from build123d import *

# Parameters (mm, degrees)
BOX002_W               = 20
BOX002_H               = 5
BOX002_DEPTH           = 10
BOX_W                  = 22.7
BOX_H                  = 12.6
BOX_DEPTH              = 17
BOX001_W               = 35
BOX001_H               = 15
BOX001_DEPTH           = 17
CUT_PLACEMENT_ANGLE    = 90
CYLINDER002_R          = 2.475
CYLINDER002_DEPTH      = 22.9
CYLINDER001_R          = 6.55
CYLINDER001_DEPTH      = 50
CUBE001_W              = 3.45
CUBE001_H              = 7.11
CUBE001_DEPTH          = 11.11
CUBE_W                 = 8.25
CUBE_H                 = 11.91
CUBE_DEPTH             = 12.91
CYLINDER_R             = 11.45
CYLINDER_DEPTH         = 45
FUSION_PLACEMENT_ANGLE = 90


with BuildPart() as cube002:
    # Box002 → Box002 (new body)
    with BuildSketch(Plane(origin=(-30, -2.5, -1), x_dir=(1, 0, 0), z_dir=(0, 0, 1))):
        with Locations((10, 2.5)):
            Rectangle(BOX002_W, BOX002_H)
    extrude(amount=BOX002_DEPTH)


with BuildPart() as cube:
    # Box → Box (new body)
    with BuildSketch(Plane.XY.offset(1)):
        with Locations((11.35, 6.3)):
            Rectangle(BOX_W, BOX_H)
    extrude(amount=BOX_DEPTH)


with BuildPart() as cut001:
    # Box001 → Box001 (new body)
    with BuildSketch(Plane(origin=(-6, -1, 0), x_dir=(1, 0, 0), z_dir=(0, 0, 1))):
        with Locations((17.5, 7.5)):
            Rectangle(BOX001_W, BOX001_H)
    extrude(amount=BOX001_DEPTH)

    # Cut: cut Cube
    add(cube.part, mode=Mode.SUBTRACT)


with BuildPart() as cut001_1:
    # Cut placement: moved
    add(cut001.part.moved(Location((-11, -6, 6))).rotate(Axis((-11, -6, 6), (0, -1, 0)), CUT_PLACEMENT_ANGLE))

    # Cut001: cut Cube002
    add(cube002.part, mode=Mode.SUBTRACT)


with BuildPart() as cylinder002:
    # cylinder002 → cylinder002 (new body)
    with BuildSketch(Plane(origin=(0, 0, 6.825), x_dir=(0, 0, -1), z_dir=(1, 0, 0))):
        Circle(CYLINDER002_R)
    extrude(amount=CYLINDER002_DEPTH)


with BuildPart() as union001:
    # cylinder001 → cylinder001 (new body)
    with BuildSketch(Plane.XY.offset(-1)):
        Circle(CYLINDER001_R)
    extrude(amount=CYLINDER001_DEPTH)

    # union001: union cylinder002
    add(cylinder002.part)


with BuildPart() as cube001:
    # cube001 → cube001 (new body)
    with BuildSketch(Plane(origin=(-1.725, -3.555, -4.6), x_dir=(1, 0, 0), z_dir=(0, 0, 1))):
        with Locations((1.725, 3.555)):
            Rectangle(CUBE001_W, CUBE001_H)
    extrude(amount=CUBE001_DEPTH)


with BuildPart() as difference:
    # cube → cube (new body)
    with BuildSketch(Plane(origin=(-4.125, -5.955, -6.455), x_dir=(1, 0, 0), z_dir=(0, 0, 1))):
        with Locations((4.125, 5.955)):
            Rectangle(CUBE_W, CUBE_H)
    extrude(amount=CUBE_DEPTH)

    # difference: cut cube001
    add(cube001.part, mode=Mode.SUBTRACT)


with BuildPart() as difference_1:
    # difference placement: moved
    add(difference.part.moved(Location((13.95, 0, 6.425))))


with BuildPart() as motor_holder:
    # cylinder → cylinder (new body)
    with BuildSketch(Plane.XY):
        Circle(CYLINDER_R)
    extrude(amount=CYLINDER_DEPTH)

    # union: union difference
    add(difference_1.part)

    # difference001: cut union001
    add(union001.part, mode=Mode.SUBTRACT)

    # Fusion: union Cut001
    add(cut001_1.part)


with BuildPart() as motor_holder_1:
    # Fusion placement: moved
    add(motor_holder.part.moved(Location((-21, 50, 0))).rotate(Axis((-21, 50, 0), (0, 0, 1)), FUSION_PLACEMENT_ANGLE))


solid = motor_holder_1.part
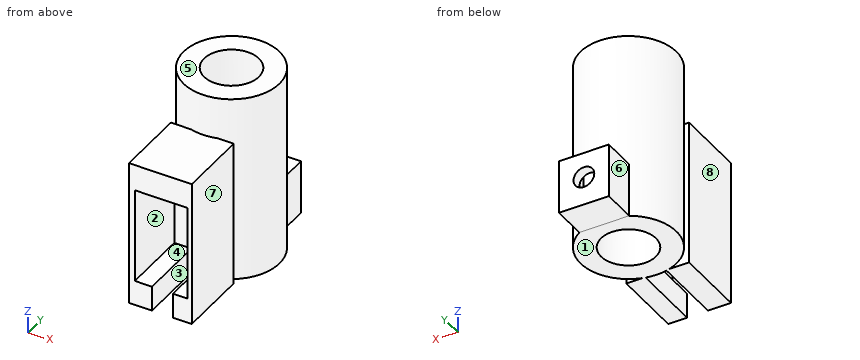
The listing builds one solid part. Answer for the finished solid, in the listing's coordinates (mm). Face numbers are marked on the shaded views. A direction names the side the tool comes from. Give positions to 0.01 mm unless a question says otherwise; leave off trailing zeros. Write each loop counter-clockwise with the first axis right and the second up, starting at its lowest first coordinate (ties: lowest second). Pieces come first, ordered by that corner, then holes. Notation, with made-up numbers: (-7.5, 45.25) -> (3.5, 45.25) arc R25 ccw to (3.5, 59.25) -> close; hole circle Ø1 at (6, -20.75). An arc over 180 degrees is marked (long way). Use a Markdown table: item, result.
(1) Flat-ended cylindrical pins translate along their axes: P1, Ø2.5, axis at y = 62.5, z = 6, coming from the +X side (3 decimals); P2, Ø13.5, axis at y = 32.5, z = 9.5, coming from the -X side; P3, Ø8, axis at y = 61, z = 27.5, coming from the -X side. Find the tip coordinate at first contact, or state that the pin passes through.
Return value:
| item | result |
|---|---|
| P1 | x = -15.045 |
| P2 | x = -29 |
| P3 | x = -30.06 |
(2) Section C-C, the plane z = 19 is taken. Determine the outline of the cut face in (x, y).
Return value:
| item | result |
|---|---|
| outline | (-29, 22) -> (-27.6, 22) -> (-27.6, 38) -> (-15, 38) -> (-15, 22) -> (-14, 22) -> (-14, 39) -> (-17.82, 39) arc R11.45 ccw (long way) to (-24.18, 39) -> (-29, 39) -> close; hole circle Ø13.1 at (-21, 50) |
(3) Section A-A, the plane y = 50 is taken. Determine the outline of the cut face in (x, z), then the cut area to 3 significant figures.
Return value:
| item | result |
|---|---|
| outline | (-32.45, 0) -> (-27.55, 0) -> (-27.55, 45) -> (-32.45, 45) -> close; (-14.45, 0) -> (-9.55, 0) -> (-9.55, 45) -> (-14.45, 45) -> close |
| area | 441 mm2 |
(4) Determine the mould class of the marked faces 1, 2 and 3 for opening direction Z: released by +Z, released by -Z, zero draft, split by the parting line, or undercut.
Return value:
| item | result |
|---|---|
| face 1 | released by -Z |
| face 2 | undercut |
| face 3 | zero draft |
(5) Section D-D, the plane y = 63 is taken. Determine the outline of the cut face in (x, z) (3 decimals), then the cut area to 3 significant figures.
Return value:
| item | result |
|---|---|
| outline | (-26.955, -0.03) -> (-15.045, -0.03) -> (-15.045, 12.88) -> (-17.445, 12.88) -> (-17.445, 1.825) -> (-24.555, 1.825) -> (-24.555, 12.88) -> (-26.955, 12.88) -> close |
| area | 75.2 mm2 |
(6) For the marked faces 4, 5, 6, 7 and 8, determine the directions among +Z, -Z, +X, -X, +Y, -Y from which every point of the face is accessible in a straight line to the end or side of a thin tool.
Return value:
| item | result |
|---|---|
| face 4 | -Y |
| face 5 | +Z, +X, -X, +Y, -Y |
| face 6 | +Z, -Z, -X, +Y |
| face 7 | +Z, -Z, +X, -Y |
| face 8 | +Z, -Z, -X, -Y |
(7) Section B-B, the plane x = -21 is taken. Give the number of separate pieces and of enclosed holes in the cut face, then the cut area to 3 significant figures.
Return value:
| item | result |
|---|---|
| separate pieces | 4 |
| enclosed holes | 0 |
| area | 564 mm2 |
(8) Find the intervals of material crossed by probe 1 along Y at (x, z) = (-15.5, 17); probe 2 along Z at (x, y) = (-21, 59); probe 3 along Y at (x, z) = (-20.75, 18), in increasing order. Write a range as from..to.
Return value:
| item | result |
|---|---|
| probe 1 | 38..39, 39.96..46.44, 53.56..60.04 |
| probe 2 | 0..4.35, 9.3..45 |
| probe 3 | 38..43.45, 56.55..61.45 |
